Source: CAD feature listing. Evaluate the final solid. Frame: model axes, mm. A direction names the side the tool comes from. Give positions to 0.01 mm unless a question says otherwise; leave off trailing zeros. Order: outer loops, then holes, each group sorted by start corner. A loop starts at its lowest first (then second) coordinate and runs counter-clockwise, first axis right, second up.
1) First-contact query: P1, Ø3, axis at y = -46.5, z = 4.5, coming from the -X side; P2, Ø2, axis at x = 40.5, z = 27, coming from the -Y side; P3, Ø8, axis at y = -36.5, z = 13, coming from the +X side. Flat tips, straight axial feed; report the tip coordinate or a pass-through.
2) Section C-C, the plane y = -15. Return loops of the section in (x, z).
3) Section B-B, the plane z = 8. Return loops of the section in (x, y), plus the area to 3 significant figures.
4) Material intervals for line 1 (X direction, y = -16, z = -1); line 2 (Z direction, x = 0, y = -46.5); line 3 (Z direction, x = 0, y = 16), sorted ascending.
5) Access query for faces 1 (the face through (-44, -30, 1)), 2 (the face through (-1, 0, -50)). Directions: +Z, -Z, +X, -X, +Y, -Y. A direction counts if a zero-diameter tool reaches every point of the face in a straight line with its end or side. Return the directions, or none.
6) Section D-D, the plane z = -35. Return loops of the section in (x, y), plus the area to 3 significant figures.
7) Section A-A, the plane x = 0. Return loops of the section in (y, z).
```python
from build123d import *

# Parameters (mm, degrees)
F0_W      = 130
F0_H      = 100
F1_DEPTH  = 30
F1_FACE_W = 130
F1_FACE_H = 100
F2_DEPTH  = 30
F3_R      = 39.856576
F3_R_2    = 33.013894
F4_DEPTH  = 30
F4_FACE_R = 33.013894
F5_DEPTH  = 60


with BuildPart() as f1:
    # F0 (on Front) → F1 (new body)
    with BuildSketch(Plane.XZ):
        Rectangle(F0_W, F0_H)
    extrude(amount=F1_DEPTH)

    # F1_face (on face) → F2 (join)
    with BuildSketch(Plane(origin=(0, 0, 0), x_dir=(1, 0, 0), z_dir=(0, 1, 0))):
        Rectangle(F1_FACE_W, F1_FACE_H)
    extrude(amount=F2_DEPTH)

    # F3 (on face) → F4 (join)
    with BuildSketch(Plane.XZ.offset(30)):
        Circle(F3_R)
        Circle(F3_R_2, mode=Mode.SUBTRACT)
    extrude(amount=F4_DEPTH)

    # F4_face (on face) → F5 (cut)
    with BuildSketch(Plane.XZ.offset(30)):
        Circle(F4_FACE_R)
    extrude(amount=-F5_DEPTH, mode=Mode.SUBTRACT)


solid = f1.part
```
From the geometry:
1. P1: stops at x = -39.74
1. P2: stops at y = -30
1. P3: stops at x = 38.83
2. outline: (-65, -50) - (65, -50) - (65, 50) - (-65, 50) - close; hole circle Ø66.03 at (0, 0)
3. outline: (-65, -30) - (-39.05, -30) - (-39.05, -60) - (-32.03, -60) - (-32.03, 30) - (-65, 30) - close; (32.03, -60) - (39.05, -60) - (39.05, -30) - (65, -30) - (65, 30) - (32.03, 30) - close
3. area: 4,380 mm2
4. line 1: x = -65 to -33, 33 to 65
4. line 2: z = -39.86 to -33.01, 33.01 to 39.86
4. line 3: z = -50 to -33.01, 33.01 to 50
5. face 1: -Y
5. face 2: -Z, +X, -X, +Y, -Y
6. outline: (-65, -30) - (-19.07, -30) - (-19.07, -60) - (19.07, -60) - (19.07, -30) - (65, -30) - (65, 30) - (-65, 30) - close
6. area: 8,940 mm2
7. outline: (-60, -39.86) - (-30, -39.86) - (-30, -50) - (30, -50) - (30, -33.01) - (-60, -33.01) - close; (-60, 33.01) - (30, 33.01) - (30, 50) - (-30, 50) - (-30, 39.86) - (-60, 39.86) - close
